```python
from build123d import *

# Parameters (mm, degrees)
F1_DEPTH = 213.8261944056
F2_R     = 92.4374796953
F3_DEPTH = 834.0718746185
F4_DEPTH = 265.7555639744
F5_DEPTH = 264.6364271641
F6_DEPTH = 25.4
F7_DEPTH = 416.5059328079
F8_DEPTH = 22.0245998353


with BuildPart() as f1:
    # F0 (on Front) → F1 (new body)
    with BuildSketch(Plane.XZ):
        Polygon((-378.5704374313, -238.2651567459), (953.7476301193, -238.2651567459), (456.0876488686, 79.1400074959), (456.0876488686, -112.8705143929), (-378.5704374313, -112.8705143929), align=None)
    extrude(amount=-F1_DEPTH)

    # F2 (on face) → F3 (join)
    with BuildSketch(Plane(origin=(456.0876488686, 0, 0), x_dir=(0, -1, 0), z_dir=(-1, 0, 0))):
        with Locations((-106.6404283047, -16.8652534485)):
            Circle(F2_R)
    extrude(amount=F3_DEPTH)

    # F4 (add): a face of the model
    f4_faces = [f1.faces().sort_by_distance(p)[0] for p in [
        (-378.5704374313, 106.9130972028, -175.5678355694),
    ]]
    extrude(f4_faces, amount=F4_DEPTH)

    # F5 (add): a face of the model
    f5_faces = [f1.faces().sort_by_distance(p)[0] for p in [
        (-377.98422575, 106.6404283047, -16.8652534485),
    ]]
    extrude(f5_faces, amount=F5_DEPTH)

    # F6 (add): a face of the model
    f6_faces = [f1.faces().sort_by_distance(p)[0] for p in [
        (-642.620652914, 106.6404283047, -16.8652534485),
    ]]
    extrude(f6_faces, amount=F6_DEPTH)

    # F7 (add): faces of the model
    f7_faces = [f1.faces().sort_by_distance(p)[0] for p in [
        (-668.020652914, 106.6404283047, -16.8652534485),
        (-644.3260014057, 106.9130972028, -175.5678355694),
    ]]
    extrude(f7_faces, amount=F7_DEPTH)

    # F8 (add): a face of the model
    f8_faces = [f1.faces().sort_by_distance(p)[0] for p in [
        (-1060.8319342136, 106.9130972028, -175.5678355694),
    ]]
    extrude(f8_faces, amount=F8_DEPTH)


solid = f1.part
```
Part model, mm, in its own coordinate system. A direction names the side the tool comes from. Round coordinates to 2 decimals unless told otherwise and drop trailing zeros. Write each loop counter-clockwise with the first axis right and the second up, starting at its lowest first coordinate (ties: lowest second). Pieces come first, ordered by that corner, then holes.
Item 1: Cut at D-D, the plane y = 49. Give the cut face in (x, z).
Results:
outline: (-1084.53, -89.13) - (456.09, -89.13) - (456.09, -112.87) - (-1082.86, -112.87) - (-1082.86, -238.27) - (953.75, -238.27) - (456.09, 79.14) - (456.09, 55.4) - (-1084.53, 55.4) - close
Item 2: Cut at B-B, the plane z = 2.5. Give the cut face in (x, y), plus the area to 3 significant figures.
Results:
outline: (-1084.53, 16.25) - (456.09, 16.25) - (456.09, 0) - (576.25, 0) - (576.25, 213.83) - (456.09, 213.83) - (456.09, 197.03) - (-1084.53, 197.03) - close
area: 304,000 mm2
Item 3: Two-plate mould, pull along Z, no slides. Class faces 1 (the cylindrical face through (-303.4, 126.7, -107.1)), 2 (the flat face through (-50, 105, -238.265)), 3 (the flat face through (456.088, 200, -16)), 4 (the flat face through (-1084.527, 108, -16)): +Z half, -Z half, draft (parallel to the pull), parting line (faces both ways), or undercut.
Results:
face 1: undercut
face 2: -Z half
face 3: undercut
face 4: draft
Item 4: Cut at C-C, the plane y = 145.5. Give the cut face in (x, z), plus the area to 3 significant figures.
Results:
outline: (-1084.53, -100.74) - (456.09, -100.74) - (456.09, -112.87) - (-1082.86, -112.87) - (-1082.86, -238.27) - (953.75, -238.27) - (456.09, 79.14) - (456.09, 67.01) - (-1084.53, 67.01) - close
area: 530,000 mm2
Item 5: Which spindle directions (+Z, -Z, +X, -X, +Y, -Y) get a long thin tool onto all of the face, cutting with end or side? Do faces 5 (the flat face through (-60, 0, -185)), 6 (the flat face through (-1082.857, 105, -175)), 7 (the flat face through (-303, 105, -112.871)). Say none if no direction does.
Results:
face 5: +Z, -Z, +X, -X, -Y
face 6: -Z, -X, +Y, -Y
face 7: -X, +Y, -Y
Item 6: Drop flat-ended pins along their axis: pin 1 Ø3 at (x, y) = (-416, 184) entering from +Z; pin 2 Ø3 at (x, y) = (92, 144) entering from +Z; pin 3 Ø1 at (x, y) = (-180, 50.5) entering from +Z. Give the stop position or say it passes through.
Results:
pin 1: stops at z = 35.96
pin 2: stops at z = 68.33
pin 3: stops at z = 56.95
Item 7: Probe L1, parallel to Z at x = -364, y = 176; L2, parallel to Z at x = -621, y = 86.5; L3, parallel to Y at x = -928, z = -55.5. List the from-to ranges inside material, lowest first.
Results:
L1: z = -238.27 to -112.87, -77.97 to 44.24
L2: z = -238.27 to -112.87, -107.08 to 73.35
L3: y = 22.66 to 190.62
Item 8: Cut at A-A, the plane x = -81.5. Give the cut face in (y, z), plus the area to 3 significant figures.
Results:
outline: (0, -238.27) - (213.83, -238.27) - (213.83, -112.87) - (0, -112.87) - close; circle Ø184.87 at (106.64, -16.87)
area: 53,700 mm2
